Autodesk Inventor part; units mm, degrees
ref_plane "YZ Plane" through (0, 0, 0) normal (1, 0, 0) x (0, 1, 0)
ref_plane "XZ Plane" through (0, 0, 0) normal (0, 1, 0) x (-1, 0, 0)
ref_plane "XY Plane" through (0, 0, 0) normal (0, 0, 1) x (1, 0, 0)
sketch "Sketch1" plane through (0, 0, 0) normal (0, 0, 1) x (1, 0, 0)
  line L0 (-90, -50) -> (90, -50)
  line L1 (90, -50) -> (90, 50)
  line L2 (90, 50) -> (-90, 50)
  line L3 (-90, 50) -> (-90, -50)
  line L4 (-90, -50) -> (90, 50) construction
  line L5 (90, -50) -> (-90, 50) construction
  point P0 (0, 0)
  dimension "d0" = 180
  dimension "d1" = 100
extrude "Extrusion1" add sketch "Sketch1" along normal blind 10
sketch "Sketch2" plane through (0, 0, 10) normal (0, 0, 1) x (1, 0, 0)
  circle A0 centre (0, 0) radius 10.5
  dimension "d4" = 21
extrude "Extrusion2" cut sketch "Sketch2" against normal through all
sketch "Sketch3" plane through (0, 0, 0) normal (0, 0, -1) x (-1, 0, 0)
  line L0 (-90, 18) -> (-78, 18)
  line L1 (-78, 18) -> (-78, 50)
  line L2 (-78, 50) -> (-90, 50)
  line L3 (-90, 50) -> (-90, 18)
  line L4 (78, 18) -> (90, 18)
  line L5 (90, 18) -> (90, 50)
  line L6 (90, 50) -> (78, 50)
  line L7 (78, 50) -> (78, 18)
  line L8 (78, -18) -> (90, -18)
  line L9 (90, -18) -> (90, -50)
  line L10 (90, -50) -> (78, -50)
  line L11 (78, -50) -> (78, -18)
  line L12 (-78, -18) -> (-90, -18)
  line L13 (-90, -18) -> (-90, -50)
  line L14 (-90, -50) -> (-78, -50)
  line L15 (-78, -50) -> (-78, -18)
  line L16 (-90, -50) -> (-90, 50)
  line L17 (-90, 50) -> (90, 50)
  line L18 (90, -50) -> (-90, -50)
  line L19 (90, 50) -> (90, -50)
  point P0 (0, 0)
  dimension "d7" = 32
  dimension "d8" = 12
  dimension "d9" = 12
  dimension "d10" = 32
  dimension "d11" = 12
  dimension "d12" = 32
  dimension "d13" = 12
  dimension "d14" = 32
extrude "Extrusion3" cut sketch "Sketch3" against normal blind 5 contours L3 L2 L1 L0 | L12 L15 L14 L13 | L6 L5 L4 L7 | L11 L8 L9 L10
sketch "Sketch4" plane through (0, 0, 10) normal (0, 0, 1) x (1, 0, 0)
  circle A0 centre (95, 45) radius 2.05
  circle A1 centre (95, -45) radius 2.05
  circle A2 centre (95, -25) radius 2.05
  circle A3 centre (95, 25) radius 2.05
  circle A4 centre (-95, 45) radius 2.05
  circle A5 centre (-95, 25) radius 2.05
  circle A6 centre (-95, -45) radius 2.05
  circle A7 centre (-95, -25) radius 2.05
  point P0 (0, 0)
hole "Hole1" at (95, 45, 10) at (95, 25, 10) at (95, -25, 10) at (95, -45, 10) at (-95, 45, 10) at (-95, 25, 10) at (-95, -25, 10) at (-95, -45, 10) direction (0, 0, -1) diameter 4.1 end through all
sketch "Sketch5" plane through (0, 0, 0) normal (0, 0, -1) x (-1, 0, 0)
  point P0 (0, 0)
sketch "Sketch6" plane through (0, 0, 0) normal (0, 0, -1) x (-1, 0, 0)
  line L0 (-10.1, -10.05) -> (10.1, -10.05)
  line L1 (10.1, -10.05) -> (10.1, 30.15)
  line L2 (10.1, 30.15) -> (-10.1, 30.15)
  line L3 (-10.1, 30.15) -> (-10.1, -10.05)
  line L4 (-10.1, -10.05) -> (10.1, 30.15) construction
  line L5 (10.1, -10.05) -> (-10.1, 30.15) construction
  point P0 (0, 0)
  point P1 (0, 10.05)
  dimension "d24" = 20.2
  dimension "d25" = 40.2
  dimension "d26" = 10.05
extrude "Extrusion4" cut sketch "Sketch6" against normal blind 5
sketch "Sketch7" plane through (0, 0, 10) normal (0, 0, 1) x (1, 0, 0)
  circle A0 centre (27.5, 12.5) radius 2.05
  circle A1 centre (27.5, -12.5) radius 2.05
  circle A2 centre (-27.5, 12.5) radius 2.05
  circle A3 centre (-27.5, -12.5) radius 2.05
  point P0 (0, 0)
hole "Hole2" at (-27.5, 12.5, 10) at (27.5, 12.5, 10) at (27.5, -12.5, 10) at (-27.5, -12.5, 10) direction (0, 0, -1) diameter 4.1 end through all
sketch "Sketch8" plane through (0, 0, 10) normal (0, 0, 1) x (1, 0, 0)
  circle A0 centre (-27.5, 12.5) radius 2.05
  circle A1 centre (27.5, 12.5) radius 2.05
  circle A2 centre (27.5, -12.5) radius 2.05
  circle A3 centre (-27.5, -12.5) radius 2.05
  circle A4 centre (-27.5, 12.5) radius 6
  circle A5 centre (27.5, 12.5) radius 6
  circle A6 centre (-27.5, -12.5) radius 6
  circle A7 centre (27.5, -12.5) radius 6
  point P0 (0, 0)
  dimension "d36" = 12
  dimension "d37" = 12
  dimension "d38" = 12
  dimension "d39" = 12
extrude "Extrusion5" cut sketch "Sketch8" against normal blind 5 contours A0 | A1 | A3 | A4 | A5 | A6 | A7
sketch "Sketch9" plane through (0, 0, 10) normal (0, 0, 1) x (1, 0, 0)
  circle A0 centre (-85, 45) radius 2.05
  circle A1 centre (-85, 25) radius 2.05
  circle A2 centre (-85, -25) radius 2.05
  circle A3 centre (-85, -45) radius 2.05
  circle A4 centre (85, 45) radius 2.05
  circle A5 centre (85, 25) radius 2.05
  circle A6 centre (85, -25) radius 2.05
  circle A7 centre (85, -45) radius 2.05
  line L0 (90, 50) -> (-90, 50)
  line L1 (-90, -50) -> (90, -50)
  line L2 (-90, 50) -> (-90, -50)
  line L3 (90, -50) -> (90, 50)
  point P0 (0, 0)
  dimension "d42" = 4.1
  dimension "d43" = 4.1
  dimension "d44" = 4.1
  dimension "d45" = 4.1
  dimension "d46" = 4.1
  dimension "d47" = 4.1
  dimension "d48" = 4.1
  dimension "d49" = 4.1
  dimension "d50" = 5
  dimension "d51" = 25
  dimension "d52" = 25
  dimension "d53" = 5
  dimension "d54" = 5
  dimension "d55" = 25
  dimension "d56" = 25
  dimension "d57" = 5
  dimension "d58" = 5
  dimension "d59" = 5
  dimension "d60" = 5
  dimension "d61" = 5
  dimension "d62" = 5
  dimension "d63" = 5
  dimension "d64" = 5
  dimension "d65" = 5
extrude "Extrusion6" cut sketch "Sketch9" against normal through all contours A0 | A1 | A2 | A3 | A4 | A5 | A6 | A7
sketch "Sketch10" plane through (0, 0, 10) normal (0, 0, 1) x (1, 0, 0)
  circle A0 centre (81, 0) radius 4.5
  circle A1 centre (-81, 0) radius 4.5
  line L0 (90, -50) -> (90, 50)
  line L1 (-90, 50) -> (-90, -50)
  point P0 (0, 0)
  dimension "d68" = 9
  dimension "d69" = 9
  dimension "d70" = 9
  dimension "d71" = 9
extrude "Extrusion7" cut sketch "Sketch10" against normal blind 10
sketch "Sketch11" plane through (0, 0, 10) normal (0, 0, 1) x (1, 0, 0)
  circle A0 centre (-10, 40) radius 2.05
  circle A1 centre (10, 40) radius 2.05
  circle A2 centre (-10, -40) radius 2.05
  circle A3 centre (10, -40) radius 2.05
  line L0 (90, 50) -> (-90, 50)
  line L1 (-90, -50) -> (90, -50)
  point P0 (0, 0)
  dimension "d74" = 4.1
  dimension "d75" = 4.1
  dimension "d76" = 4.1
  dimension "d77" = 4.1
  dimension "d78" = 10
  dimension "d79" = 10
  dimension "d80" = 10
  dimension "d81" = 10
  dimension "d82" = 10
  dimension "d83" = 10
  dimension "d84" = 10
  dimension "d85" = 10
extrude "Extrusion8" cut sketch "Sketch11" against normal blind 10
sketch "Sketch12" plane through (0, 0, 10) normal (0, 0, 1) x (1, 0, 0)
  circle A0 centre (-10, 40) radius 2.05
  circle A1 centre (10, 40) radius 2.05
  circle A2 centre (-10, -40) radius 2.05
  circle A3 centre (10, -40) radius 2.05
  circle A4 centre (10, 40) radius 5
  circle A5 centre (-10, 40) radius 5
  circle A6 centre (10, -40) radius 5
  circle A7 centre (-10, -40) radius 5
  point P0 (0, 0)
  dimension "d88" = 10
  dimension "d89" = 10
  dimension "d90" = 10
  dimension "d91" = 10
extrude "Extrusion9" cut sketch "Sketch12" against normal blind 5 contours A0 | A1 | A2 | A3 | A4 | A5 | A6 | A7
sketch "Sketch13" plane through (0, 0, 10) normal (0, 0, 1) x (1, 0, 0)
  circle A0 centre (10, -40) radius 5
  circle A1 centre (10, 40) radius 5
  circle A2 centre (-10, -40) radius 5
  circle A3 centre (-10, 40) radius 5
  circle A4 centre (81, 0) radius 4.5
  circle A5 centre (-81, 0) radius 4.5
  circle A6 centre (-85, -25) radius 2.05
  circle A7 centre (85, -25) radius 2.05
  circle A8 centre (85, 25) radius 2.05
  circle A9 centre (-85, 25) radius 2.05
  circle A10 centre (-85, -45) radius 2.05
  circle A11 centre (85, -45) radius 2.05
  circle A12 centre (85, 45) radius 2.05
  circle A13 centre (-85, 45) radius 2.05
  circle A14 centre (27.5, -12.5) radius 6
  circle A15 centre (27.5, 12.5) radius 6
  circle A16 centre (-27.5, -12.5) radius 6
  circle A17 centre (-27.5, 12.5) radius 6
  circle A18 centre (0, 0) radius 10.5
  line L0 (90, -50) -> (90, 50)
  line L1 (90, 50) -> (-90, 50)
  line L2 (-90, 50) -> (-90, -50)
  line L3 (-90, -50) -> (90, -50)
extrude "Extrusion10" add sketch "Sketch13" along normal blind 5
sketch "Sketch14" plane through (-10, 40, 5) normal (0, 0, 1) x (1, 0, 0)
  circle A0 centre (0, 0) radius 2.05
  circle A1 centre (0, 0) radius 5
  circle A2 centre (20, 0) radius 2.05
  circle A3 centre (20, 0) radius 5
  circle A4 centre (-17.5, -27.5) radius 2.05
  circle A5 centre (-17.5, -27.5) radius 6
  circle A6 centre (37.5, -27.5) radius 2.05
  circle A7 centre (37.5, -27.5) radius 6
  circle A8 centre (-17.5, -52.5) radius 2.05
  circle A9 centre (-17.5, -52.5) radius 6
  circle A10 centre (37.5, -52.5) radius 6
  circle A11 centre (37.5, -52.5) radius 2.05
  circle A12 centre (0, -80) radius 2.05
  circle A13 centre (0, -80) radius 5
  circle A14 centre (20, -80) radius 2.05
  circle A15 centre (20, -80) radius 5
  point P0 (10, -40)
extrude "Extrusion11" add sketch "Sketch14" along normal blind 5
fillet "Fillet1" radius 1 12 edges at (90, 50, 10) (90, -50, 10) (-90, -50, 10) (-90, 50, 10) (90, -18, 2.5) (90, 18, 2.5) (78, -50, 2.5) (78, 50, 2.5) (-90, 18, 2.5) (-90, -18, 2.5) (-78, -50, 2.5) (-78, 50, 2.5)
properties part number "gripper_base" material "ABS Plastic"
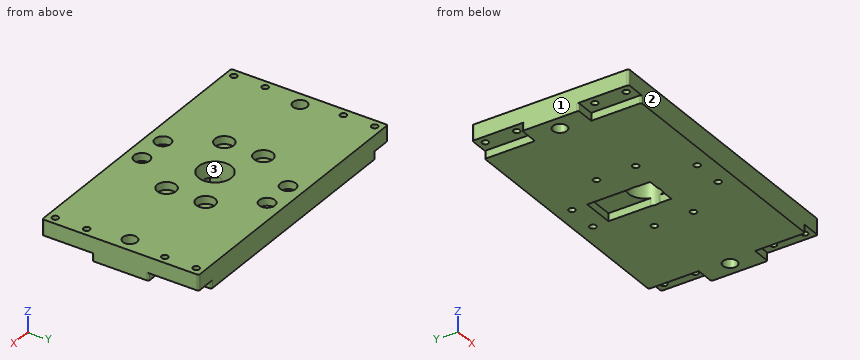
Here's how the part is built. I have some questions about the finished solid (model axes, mm). Face numbers are marked on the shaded views. Give positions to 0.01 mm unless a question says otherwise; leave off trailing zeros. Order: outer loops, then holes, each group sorted by start corner. A loop starts at its lowest first (then second) coordinate and runs counter-clockwise, first axis right, second up. Notation, with made-up numbers: (45, -30.75) -> (95, -30.75) arc R28 cw to (95, 6.25) -> close; hole circle Ø8 at (-3.5, -12). An arc over 180 degrees is marked (long way). Use CSV: the item, a comma, the result in double quotes. Start each with the question number.
Item 1: Thinking about a two-plate mould opening in Y: for the marked faces 1, 2 and 3, which applies, pulls with the +Y half, pulls with the -Y half, needs draft (parallel to the pull), parting line crosses it, or undercut?
Item 2: Suppose I cut it at C-C (y = -40). List the corners of the cut face in (x, z) for me.
Item 3: I'm going to push flat-ended pins straight in: P1, Ø6, axis at x = 5, y = 13.5, coming from the -Z side; P2, Ø6, axis at x = 10, y = -40, coming from the +Z side. Where does each tip first touch, or does it pass through?
Item 4: If I drill on probe 1 along Y at (x, z) = (27.5, 12.5); probe 2 along Y at (x, z) = (27.5, 7.75); probe 3 along X at (y, z) = (-12.5, 4.25), over which ranges is the centre line in solid material (lowest first)? Write a range as [from, to].
Item 5: Suppose I cut it at A-A (z = 12.5). Give the number of separate pieces and of enclosed holes in the cut face, and give its area (3 significant figures).
Item 6: Suppose I cut it at B-B (x = 0). List the corners of the cut face in (y, z) for me, and give its area (3 significant figures).
Answer block:
1,face 1,"needs draft"
1,face 2,"pulls with the -Y half"
1,face 3,"undercut"
2,outline,"(-90, 5) -> (-78, 5) -> (-78, 0) -> (-12.05, 0) -> (-12.05, 10) -> (-15, 10) -> (-15, 15) -> (-90, 15) -> close; (-7.95, 0) -> (7.95, 0) -> (7.95, 10) -> (5, 10) -> (5, 15) -> (-5, 15) -> (-5, 10) -> (-7.95, 10) -> close; (12.05, 0) -> (78, 0) -> (78, 5) -> (90, 5) -> (90, 15) -> (15, 15) -> (15, 10) -> (12.05, 10) -> close"
3,P1,"stops at z = 5"
3,P2,"stops at z = 10"
4,probe 1,"y = [-50, -18.5], [-6.5, 6.5], [18.5, 50]"
4,probe 2,"y = [-50, -14.55], [-10.45, 10.45], [14.55, 50]"
4,probe 3,"x = [-90, -29.55], [-25.45, 25.45], [29.55, 90]"
5,separate pieces,"1"
5,enclosed holes,"19"
5,area,"16,700 mm^2"
6,outline,"(-50, 0) -> (-10.5, 0) -> (-10.5, 15) -> (-50, 15) -> close; (10.5, 5) -> (30.15, 5) -> (30.15, 0) -> (50, 0) -> (50, 15) -> (10.5, 15) -> close"
6,area,"1,090 mm^2"
